Could you check a few things on this model? Use its own coordinates, in mm. A direction names the side the tool comes from. Give positions to 0.01 mm unless a question says otherwise; leave off trailing zeros. Loops run counter-clockwise (first coordinate to the right, second up) from the corner with the lowest first, then second, coordinate; pieces in that order, holes last. Notation, with made-up numbers: M 59.25,-19 L 95.25,-19 A37 cw 95.25,20 Z; hole C 71,15 d1. An arc over 180 degrees is marked long. Return JSON: item names as keys, results as strings. Group by question number.
1. If we section it at B-B (x = -21): Write out the boundary of the cut face in (y, z).
2. For faces 1 (the cylindrical face through (-19.41, 121.53, -1.45)), 2 (the flat face through (-19, 114, 0)), which set-ups out of +Z, -Z, +X, -X, +Y, -Y let a thin tool reach every point of the face, with its end or its side?
3. Please list where these lines run through material, in increasing order: line 1 (Z direction, x = -11.5, y = 122); line 2 (X direction, y = 120.75, z = -1.75); line 3 (Y direction, x = -21.25, z = -2.5).
4. If we section it at C-C (z = -1): Write out the boundary of the cut face in (x, y), plus the area to 3 significant figures.
5. If we section it at A-A (y = 119): Write out the boundary of the cut face in (x, z).
6. If we section it at D-D (x = -15.5): Write out the boundary of the cut face in (y, z).
7. For pin 1 (12 mm diameter, centred on x = -10.5, y = 116, fed in from -Z); pin 2 (1.5 mm diameter, centred on y = 110.5, z = 1, fed in from +X), each with a flat end and sliding along its axis, tell me the tip position at first contact or that it passes through.
Autodesk Inventor part; units mm, degrees
ref_plane "YZ Plane" through (0, 0, 0) normal (1, 0, 0) x (0, 1, 0)
ref_plane "XZ Plane" through (0, 0, 0) normal (0, 1, 0) x (-1, 0, 0)
ref_plane "XY Plane" through (0, 0, 0) normal (0, 0, 1) x (1, 0, 0)
ref_plane "Work Plane1" through (0, 0, 0) normal (0, 0, 1) x (1, 0, 0)
sketch "Sketch1" plane through (0, 0, 0) normal (0, 0, 1) x (1, 0, 0)
  circle A0 centre (-19.0766, 119) radius 8
  circle A1 centre (-19.0766, 119) radius 4.5
  circle A2 centre (-19.0766, 119) radius 2.55
  point P0 (0, 0)
  dimension "d0" = 9
  dimension "d1" = 5.1
extrude "Extrusion1" add sketch "Sketch1" against normal blind 5 contours A1
sketch "Sketch2" plane through (-19.0766, 119, 0) normal (0, 0, 1) x (1, 0, 0)
  circle A0 centre (0, 0) radius 2.55
  circle A1 centre (0, 0) radius 11
  point P0 (19.0766, -119)
  dimension "d4" = 22
extrude "Extrusion2" add sketch "Sketch2" along normal blind 2
properties part number "13_Fluorescence_Arm_LEDholder"
Answer:
{
 "1": {"outline": "M 108.17,0 L 114.93,0 L 114.93,-5 L 117.33,-5 L 117.33,2 L 108.17,2 Z; M 120.67,-5 L 123.07,-5 L 123.07,0 L 129.83,0 L 129.83,2 L 120.67,2 Z"},
 "2": {"face 1": "+Z, -Z", "face 2": "-Z"},
 "3": {"line 1": "z = 0 to 2", "line 2": "x = -23.22 to -20.93, -17.22 to -14.93", "line 3": "y = 115.06 to 117.67, 120.33 to 122.94"},
 "4": {"outline": "C -19.08,119 d9; hole C -19.08,119 d5.1", "area": "43.2 mm²"},
 "5": {"outline": "M -30.08,0 L -23.58,0 L -23.58,-5 L -21.63,-5 L -21.63,2 L -30.08,2 Z; M -16.53,-5 L -14.58,-5 L -14.58,0 L -8.08,0 L -8.08,2 L -16.53,2 Z"},
 "6": {"outline": "M 108.6,0 L 116.27,0 L 116.27,-5 L 121.73,-5 L 121.73,0 L 129.4,0 L 129.4,2 L 108.6,2 Z"},
 "7": {"pin 1": "stops at z = -5", "pin 2": "stops at x = -11.27"}
}
